```python
from build123d import *

# Parameters (mm, degrees)
CROQUIS1_R              = 2.25
CROQUIS1_R_2            = 3
CROQUIS1_R_3            = 1.5
CROQUIS1_R_4            = 2.249997567
SALIENTE_EXTRUIR1_DEPTH = 2.5
CROQUIS2_R              = 1.5
SALIENTE_EXTRUIR2_DEPTH = 2.5
CORTAR_EXTRUIR3_START   = -2.5
CROQUIS3_W              = 193.648563709
CROQUIS3_H              = 122.889896528
CORTAR_EXTRUIR3_DEPTH   = 2.5


with BuildPart() as part:
    # Croquis1 → Saliente-Extruir1 (new body)
    with BuildSketch(Plane.XY):
        with BuildLine():
            Line((-29.502526327, -44.949972179), (-23.17778065, -37.243838032))
            ThreePointArc((-23.17778065, -37.243838032), (-18.839723212, -32.444384768), (-14.046056443, -28.099933953))
            ThreePointArc((-14.046056443, -28.099933953), (-12.991422185, -27.658257217), (-11.867164621, -27.866527921))
            ThreePointArc((-11.867164621, -27.866527921), (-11.203313373, -28.112469078), (-10.500314, -28.196))
            Line((-10.500314, -28.196), (10.499686, -28.196))
            ThreePointArc((10.499686, -28.196), (11.203007921, -28.112542722), (11.867164264, -27.866528101))
            ThreePointArc((11.867164264, -27.866528101), (12.991422421, -27.658256674), (14.046057406, -28.099933523))
            ThreePointArc((14.046057406, -28.099933523), (18.839775902, -32.444337151), (23.177889012, -37.243749049))
            Line((23.177889012, -37.243749049), (29.502526012, -44.949972049))
            ThreePointArc((29.502526012, -44.949972049), (40.113877497, -46.255199126), (41.931739547, -35.719556022))
            Line((41.931739547, -35.719556022), (21.72923101, -5.566101046))
            ThreePointArc((21.72923101, -5.566101046), (20.036969431, -9.5e-08), (21.729230693, 5.566100954))
            Line((21.729230693, 5.566100954), (41.931739693, 35.719555954))
            ThreePointArc((41.931739693, 35.719555954), (40.113877277, 46.255198335), (29.502526336, 44.949972165))
            Line((29.502526336, 44.949972165), (23.17778065, 37.243838007))
            ThreePointArc((23.17778065, 37.243838007), (18.839723212, 32.444384742), (14.046056443, 28.099933927))
            ThreePointArc((14.046056443, 28.099933927), (12.991421988, 27.658257139), (11.867164252, 27.866528027))
            ThreePointArc((11.867164252, 27.866528027), (11.203313175, 28.112469073), (10.500314, 28.195999974))
            Line((10.500314, 28.195999974), (-10.500314, 28.195999974))
            ThreePointArc((-10.500314, 28.195999974), (-11.203313178, 28.112469098), (-11.867164264, 27.866528075))
            ThreePointArc((-11.867164264, 27.866528075), (-12.991422421, 27.658256648), (-14.046057406, 28.099933497))
            ThreePointArc((-14.046057406, 28.099933497), (-18.839775902, 32.444337126), (-23.177889012, 37.243749023))
            Line((-23.177889012, 37.243749023), (-29.502526012, 44.949972023))
            ThreePointArc((-29.502526012, 44.949972023), (-40.146302424, 46.230987494), (-41.886340556, 35.652554517))
            ThreePointArc((-41.886340556, 35.652554517), (-41.288874902, 25.337679941), (-50.13550001, 20.000000021))
            Line((-50.13550001, 20.000000021), (-97.31807601, 20.000000021))
            ThreePointArc((-97.31807601, 20.000000021), (-99.1994919, 19.554558541), (-100.681450855, 18.312809163))
            add(Edge.make_bspline(
                [(-107.31807554, 2.1e-08), (-107.252414123, 7.059743944), (-104.975710329, 13.164639039), (-100.681450855, 18.312809163)],
                knots=[0, 0, 0, 0, 1, 1, 1, 1], degree=3))
            add(Edge.make_bspline(
                [(-107.31807554, 2.1e-08), (-107.252414123, -7.059743902), (-104.975710329, -13.164638997), (-100.681450855, -18.312809121)],
                knots=[0, 0, 0, 0, 1, 1, 1, 1], degree=3))
            ThreePointArc((-100.681450855, -18.312809121), (-99.19949186, -19.554558345), (-97.31807601, -19.9999997))
            Line((-97.31807601, -19.9999997), (-50.13550001, -19.9999997))
            ThreePointArc((-50.13550001, -19.9999997), (-41.288874902, -25.33767962), (-41.886340556, -35.652554196))
            ThreePointArc((-41.886340556, -35.652554196), (-40.146302646, -46.230987042), (-29.502526327, -44.949972179))
        make_face()
        with Locations((-25.371621, 27.641642)):
            Circle(CROQUIS1_R, mode=Mode.SUBTRACT)
        with Locations((-35.493242035, 40.033284004)):
            Circle(CROQUIS1_R, mode=Mode.SUBTRACT)
        with Locations((-35.49324201, -40.0332837)):
            Circle(CROQUIS1_R, mode=Mode.SUBTRACT)
        with Locations((15.25, -15.25)):
            Circle(CROQUIS1_R_2, mode=Mode.SUBTRACT)
        with Locations((35.493242035, -40.03328403)):
            Circle(CROQUIS1_R, mode=Mode.SUBTRACT)
        with Locations((-15.25, 15.25)):
            Circle(CROQUIS1_R_2, mode=Mode.SUBTRACT)
        with Locations((-25.371621, -27.641642)):
            Circle(CROQUIS1_R, mode=Mode.SUBTRACT)
        with Locations((-35.318076, 15.5)):
            Circle(CROQUIS1_R_3, mode=Mode.SUBTRACT)
        with Locations((25.371621, -27.641642)):
            Circle(CROQUIS1_R, mode=Mode.SUBTRACT)
        with Locations((-15.25, -15.25)):
            Circle(CROQUIS1_R_2, mode=Mode.SUBTRACT)
        with Locations((-97.318076, 15.5)):
            Circle(CROQUIS1_R_3, mode=Mode.SUBTRACT)
        with Locations((15.25, 15.25)):
            Circle(CROQUIS1_R_2, mode=Mode.SUBTRACT)
        with Locations((-35.318076, -15.5)):
            Circle(CROQUIS1_R_3, mode=Mode.SUBTRACT)
        with Locations((25.371621, 27.641642)):
            Circle(CROQUIS1_R, mode=Mode.SUBTRACT)
        with Locations((-97.318076, -15.5)):
            Circle(CROQUIS1_R_3, mode=Mode.SUBTRACT)
        with Locations((35.493241695, 40.03328329)):
            Circle(CROQUIS1_R_4, mode=Mode.SUBTRACT)
        with BuildLine():
            Line((10.499686, -24.196), (-10.500314, -24.196))
            ThreePointArc((-10.500314, -24.196), (-11.500314, -25.196), (-10.500314, -26.196))
            Line((-10.500314, -26.196), (10.499686, -26.196))
            ThreePointArc((10.499686, -26.196), (11.499686, -25.196), (10.499686, -24.196))
        make_face(mode=Mode.SUBTRACT)
        with BuildLine():
            Line((10.499686, 24.196), (-10.500314, 24.196))
            ThreePointArc((-10.500314, 24.196), (-11.500314, 25.196), (-10.500314, 26.196))
            Line((-10.500314, 26.196), (10.499686, 26.196))
            ThreePointArc((10.499686, 26.196), (11.499686, 25.196), (10.499686, 24.196))
        make_face(mode=Mode.SUBTRACT)
        with BuildLine():
            Line((-85.514124, -4.165983), (-47.669779, -4.165983))
            ThreePointArc((-47.669779, -4.165983), (-45.229883846, -6.121043634), (-46.606106368, -8.928419991))
            ThreePointArc((-46.606106368, -8.928419991), (-47.664637652, -9.309528853), (-48.775706549, -9.486329166))
            ThreePointArc((-48.775706549, -9.486329166), (-65.20554454, -10.947799765), (-81.54268179, -13.222314916))
            ThreePointArc((-81.54268179, -13.222314916), (-86.502756567, -11.787005843), (-88.511039815, -7.029984473))
            ThreePointArc((-88.511039815, -7.029984473), (-87.586803958, -4.997112835), (-85.514124, -4.165983))
        make_face(mode=Mode.SUBTRACT)
        with BuildLine():
            Line((-85.514123843, 4.165983), (-47.669779, 4.165983))
            ThreePointArc((-47.669779, 4.165983), (-45.229893438, 6.121044064), (-46.606108087, 8.928416245))
            ThreePointArc((-46.606108087, 8.928416245), (-47.664639263, 9.309527068), (-48.775708446, 9.48632916))
            ThreePointArc((-48.775708446, 9.48632916), (-65.205546063, 10.947798842), (-81.542682989, 13.222313035))
            ThreePointArc((-81.542682989, 13.222313035), (-86.502748912, 11.786999538), (-88.511029539, 7.029984958))
            ThreePointArc((-88.511029539, 7.029984958), (-87.586797502, 4.997116506), (-85.514123843, 4.165983))
        make_face(mode=Mode.SUBTRACT)
    extrude(amount=SALIENTE_EXTRUIR1_DEPTH)

    # Croquis2 → Saliente-Extruir2 (add)
    with BuildSketch(Plane.XY.offset(2.5)):
        with BuildLine():
            Line((-50.13550001, 20.000000021), (-30.318076, 20.000000021))
            Line((-30.318076, 20.000000021), (-30.318076, -19.9999997))
            Line((-30.318076, -19.9999997), (-50.13550001, -19.9999997))
            Line((-50.13550001, -19.9999997), (-97.31807601, -19.9999997))
            ThreePointArc((-97.31807601, -19.9999997), (-99.19949186, -19.554558345), (-100.681450855, -18.312809121))
            add(Edge.make_bspline(
                [(-107.31807554, 2.1e-08), (-107.252414123, -7.059743902), (-104.975710329, -13.164638997), (-100.681450855, -18.312809121)],
                knots=[0, 0, 0, 0, 1, 1, 1, 1], degree=3))
            add(Edge.make_bspline(
                [(-100.681450855, 18.312809163), (-104.975710329, 13.164639039), (-107.252414123, 7.059743944), (-107.31807554, 2.1e-08)],
                knots=[0, 0, 0, 0, 1, 1, 1, 1], degree=3))
            ThreePointArc((-100.681450855, 18.312809163), (-99.1994919, 19.554558541), (-97.31807601, 20.000000021))
            Line((-97.31807601, 20.000000021), (-50.13550001, 20.000000021))
        make_face()
        with Locations((-35.318076, 15.5)):
            Circle(CROQUIS2_R, mode=Mode.SUBTRACT)
        with Locations((-35.318076, -15.5)):
            Circle(CROQUIS2_R, mode=Mode.SUBTRACT)
        with Locations((-97.318076, -15.5)):
            Circle(CROQUIS2_R, mode=Mode.SUBTRACT)
        with Locations((-97.318076, 15.5)):
            Circle(CROQUIS2_R, mode=Mode.SUBTRACT)
    extrude(amount=SALIENTE_EXTRUIR2_DEPTH)

    # Croquis3 → Cortar-Extruir3 (cut)
    with BuildSketch(Plane.XY.offset(2.5).offset(CORTAR_EXTRUIR3_START)):
        with Locations((-31.186912947, -1.649898241)):
            Rectangle(CROQUIS3_W, CROQUIS3_H)
    extrude(amount=CORTAR_EXTRUIR3_DEPTH, mode=Mode.SUBTRACT)


solid = part.part
```
Source: CAD feature listing. Evaluate the final solid. Frame: model axes, mm. Round coordinates to 2 decimals unless told otherwise and drop trailing zeros. Use a Markdown table: item, result. Add a question column.
1. Mould query, pull axis Y, two halves, no side actions, for faces 1 (the cylindrical face through (-99.175, -19.567, 3.732)), 2 (the flat face through (-68, 0, 5)), 3 (the cylindrical face through (-36.817, 15.566, 3.732)). Classes: pulls with the +Y half, pulls with the -Y half, needs draft (parallel to the pull), parting line crosses it, or undercut.
2. Section query A-A on z = 3.5. Give the number of separate pieces and of enclosed holes in the cut face, then the cut area to 3 significant figures.
3. Line query: line 1 (X direction, y = -15.5, z = 3.75); line 2 (Y direction, x = -36, z = 4.3); line 3 (X direction, y = -5.5, z = 4). Output: solid intervals per line, ascending.
4. Contact query for a flat-ended pin moving along its axis: P1, Ø2.5, axis at x = -97.32, y = 15.5, coming from the +Z side. Output: stop coordinate, or through.
Reported:
| question | item | result |
|---|---|---|
| 1 | face 1 | pulls with the -Y half |
| 1 | face 2 | needs draft |
| 1 | face 3 | undercut |
| 2 | separate pieces | 1 |
| 2 | enclosed holes | 4 |
| 2 | area | 2,950 mm² |
| 3 | line 1 | x = -102.76 to -98.82, -95.82 to -36.82, -33.82 to -30.32 |
| 3 | line 2 | y = -20 to -16.84, -14.16 to 14.16, 16.84 to 20 |
| 3 | line 3 | x = -106.79 to -30.32 |
| 4 | P1 | passes through |
